Geometry check sheet. Reference: drawing and pictorial views, mm from the part's lowest x, y, z. A direction names the side the tool comes from. Round coordinates to 2 decimals unless told otherwise and drop trailing zeros. Loops run counter-clockwise (first coordinate to the right, second up) from the corner with the lowest first, then second, coordinate; pieces in that order, holes last. Notation, with made-up numbers: (34.25, -26.5) -> (55.25, -26.5) arc R23 cw to (55.25, -9.5) -> close; hole circle Ø11 at (-17, 47). An arc over 180 degrees is marked (long way). Use one line per item in the form item = value. Start each with the question number.
(1) Material ranges on probe 1 along X at (y, z) = (45.5, 56); probe 2 along X at (y, z) = (25, 37); probe 3 along X at (y, z) = (51, 36), recorded low to high. Write a range as [from, to].
(2) Sectioned sample at D-D (z = 16.5). Record the cut outline in (x, y), and give its area (3 significant figures).
(3) Set-up check for the marked faces 4 and 5: record each of +Z, -Z, +X, -X, +Y, -Y from which the full face is reachable in a straight line by a thin tool's end or side.
(4) Sectioned sample at A-A (y = 34). Record the cut outline in (x, z), and give its area (3 significant figures).
(5) Sectioned sample at C-C (x = 23.5). Record the cut outline in (y, z).
(6) Draft check along X on the marked faces 1, 2 and 3. Enter one of: released by +X, released by -X, zero draft, split by the parting line, or undercut.
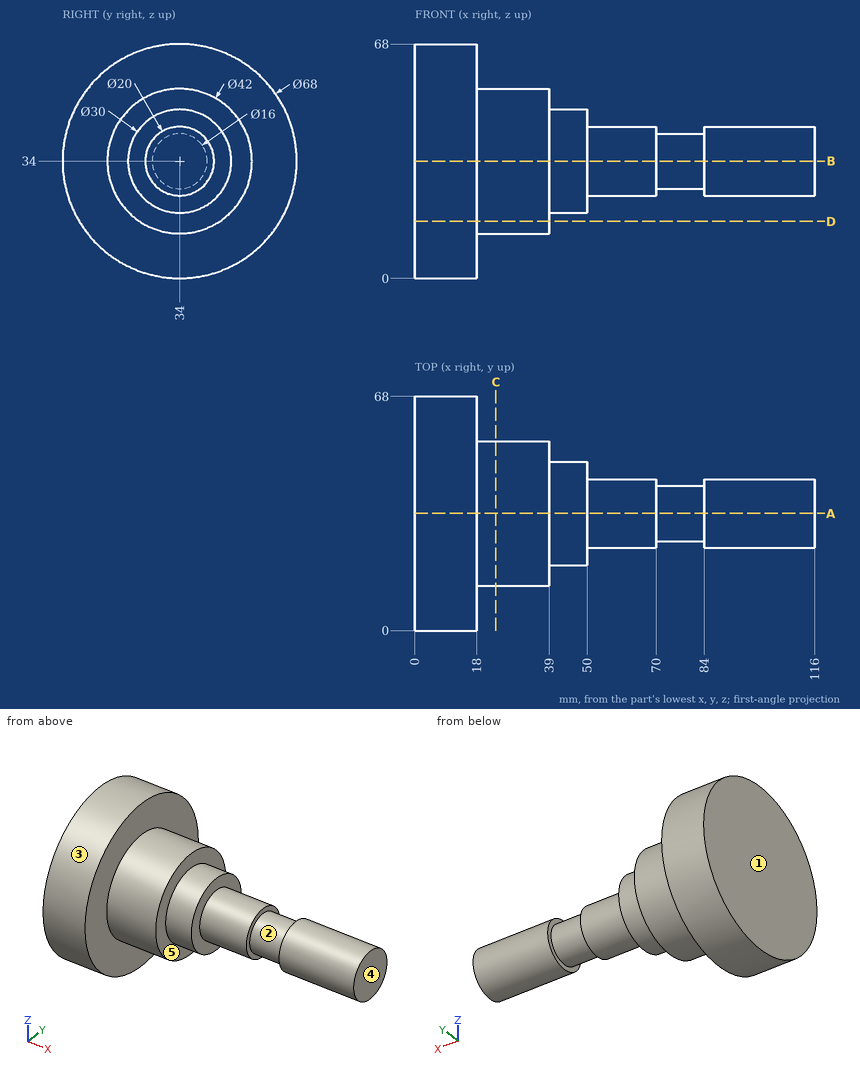
Checks:
q1.probe_1 = [0, 18]
q1.probe_2 = [0, 70], [84, 116]
q1.probe_3 = [0, 39]
q2.outline = (0, 4.85) -> (18, 4.85) -> (18, 22.39) -> (39, 22.39) -> (39, 45.61) -> (18, 45.61) -> (18, 63.15) -> (0, 63.15) -> close
q2.area = 1,540 mm2
q3.face_4 = +Z, -Z, +X, +Y, -Y
q3.face_5 = +X
q4.outline = (0, 0) -> (18, 0) -> (18, 13) -> (39, 13) -> (39, 19) -> (50, 19) -> (50, 24) -> (70, 24) -> (70, 26) -> (84, 26) -> (84, 24) -> (116, 24) -> (116, 44) -> (84, 44) -> (84, 42) -> (70, 42) -> (70, 44) -> (50, 44) -> (50, 49) -> (39, 49) -> (39, 55) -> (18, 55) -> (18, 68) -> (0, 68) -> close
q4.area = 3,700 mm2
q5.outline = circle Ø42 at (34, 34)
q6.face_1 = released by -X
q6.face_2 = undercut
q6.face_3 = zero draft
